The listing builds one solid part. Answer for the finished solid, in the listing's coordinates (mm). Face numbers are marked on the shaded views. A direction names the side the tool comes from. Give positions to 0.01 mm unless a question says otherwise; leave off trailing zeros. Loops run counter-clockwise (first coordinate to the right, second up) from the corner with the lowest first, then second, coordinate; pieces in that order, holes last. Notation, with made-up numbers: M 32,-24.5 L 37,-24.5 A26 ccw 37,9.5 Z; hole C 1.25,58.25 d4. An arc over 180 degrees is marked long. One line per item, written item: value. Start each with the question number.
Q1. Consider L1, parallel to Z at x = 36.5, y = -2.25; L2, parallel to X at y = 0.75, z = 2; L3, parallel to X at y = 1.5, z = 4.5. Determine where each line is inside the solid, lowest interval first.
Q2. A cutting plane is placed at C-C, the plane z = 10.75. Determine the outline of the cut face in (x, y), and give its area (3 significant figures).
Q3. A cutting plane is placed at A-A, the plane y = 0. Determine the outline of the cut face in (x, z).
Q4. A cutting plane is placed at D-D, the plane x = 13.5. Determine the outline of the cut face in (y, z), and give its area (3 significant figures).
Q5. For the marked faces 1 and 2, determine the directions among +Z, -Z, +X, -X, +Y, -Y from which every point of the face is accessible in a straight line to the end or side of a thin tool.
Q6. A cutting plane is placed at B-B, the plane z = 1.5. Determine the outline of the cut face in (x, y).
Autodesk Inventor part; units mm, degrees
ref_plane "YZ Plane" through (0, 0, 0) normal (1, 0, 0) x (0, 1, 0)
ref_plane "XZ Plane" through (0, 0, 0) normal (0, 1, 0) x (-1, 0, 0)
ref_plane "XY Plane" through (0, 0, 0) normal (0, 0, 1) x (1, 0, 0)
sketch "Boceto1" plane through (0, 0, 0) normal (0, 0, 1) x (1, 0, 0)
  line L0 (-13.0068, 0) -> (66.9932, 0) construction
  line L1 (-13.0068, -3.5) -> (66.9932, -3.5)
  line L2 (66.9932, 3.5) -> (-13.0068, 3.5)
  arc A0 (-13.0068, 3.5) -> (-13.0068, -3.5) centre (-13.0068, 0) ccw
  arc A1 (66.9932, -3.5) -> (66.9932, 3.5) centre (66.9932, 0) ccw
  circle A2 centre (66.9932, 0) radius 2
  point P0 (0, 0)
  point P1 (26.9932, 0)
  dimension "d0" = 80
  dimension "d1" = 7
  dimension "d2" = 4
extrude "Extrusión1" add sketch "Boceto1" along normal blind 5
sketch "Boceto3" plane through (0, 0, 5) normal (0, 0, 1) x (1, 0, 0)
  line L0 (66.9932, 3.5) -> (-13.0068, 3.5)
  circle A0 centre (-13.0068, 0) radius 3.5
  point P0 (0, 0)
extrude "Extrusión3" add sketch "Boceto3" along normal blind 7
properties part number "L3" material "Aluminio 6061"
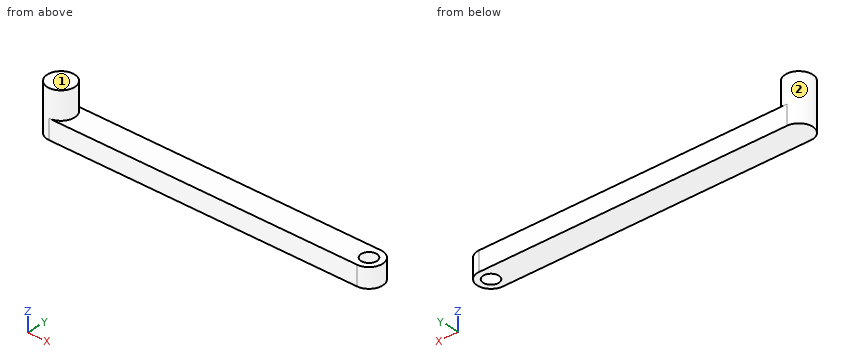
Answer block:
1. L1: 0 to 5
1. L2: -16.43 to 65.14, 68.85 to 70.41
1. L3: -16.17 to 65.67, 68.32 to 70.16
2. outline: C -13.01,0 d7
2. area: 38.5 mm^2
3. outline: M -16.51,0 L 64.99,0 L 64.99,5 L -9.51,5 L -9.51,12 L -16.51,12 Z; M 68.99,0 L 70.49,0 L 70.49,5 L 68.99,5 Z
4. outline: M -3.5,0 L 3.5,0 L 3.5,5 L -3.5,5 Z
4. area: 35.0 mm^2
5. face 1: +Z, +X, -X, +Y, -Y
5. face 2: +Z
6. outline: M -13.01,-3.5 L 66.99,-3.5 A3.5 ccw 66.99,3.5 L -13.01,3.5 A3.5 ccw Z; hole C 66.99,0 d4
